Verification items for the finished model (mm, model axes). Face numbers are marked on the shaded views. A direction names the side the tool comes from. Round coordinates to 2 decimals unless told otherwise and drop trailing zeros. Loops run counter-clockwise (first coordinate to the right, second up) from the corner with the lowest first, then second, coordinate; pieces in that order, holes last. Notation, with made-up numbers: M -9.75,42.25 L 28.25,42.25 A36 ccw 28.25,81.25 Z; hole C 23,18.25 d5. An arc over 180 degrees is marked long. Answer as CSV lines item,"result".
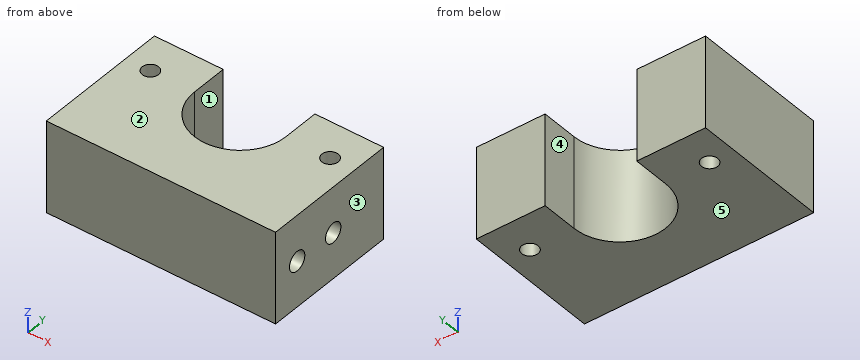
```python
from build123d import *

# Parameters (mm, degrees)
SKETCH1_W                 = 12.7
SKETCH1_H                 = 19.05
BASE_DEPTH                = 31.75
MOTORSLOT_DEPTH           = 40.144028919
MOTORHOLES_D              = 2.2606
F_6_32_TAPPED_HOLE1_D     = 2.7051
F_6_32_TAPPED_HOLE1_DEPTH = 8.382
F_6_32_TAPPED_HOLE1_TIP   = 0.81269403


with BuildPart() as part:
    # Sketch1 → Base (new body)
    with BuildSketch(Plane(origin=(0, 0, 0), x_dir=(0, 0, -1), z_dir=(1, 0, 0))):
        with Locations((6.35, 9.525)):
            Rectangle(SKETCH1_W, SKETCH1_H)
    extrude(amount=-BASE_DEPTH)

    # Sketch5 → MotorSlot (cut, through all)
    with BuildSketch(Plane(origin=(0, 0, -12.7), x_dir=(-1, 0, 0), z_dir=(0, 0, -1))):
        with BuildLine():
            Line((22.225, 19.05), (22.225, 13.97))
            ThreePointArc((22.225, 13.97), (15.875, 7.62), (9.525, 13.97))
            Line((9.525, 13.97), (9.525, 19.05))
            ThreePointArc((9.525, 19.05), (15.875, 25.4), (22.225, 19.05))
        make_face()
    extrude(amount=-MOTORSLOT_DEPTH, mode=Mode.SUBTRACT)

    # MotorHoles (through all)
    with Locations(Plane(origin=(0, 0, -12.7), x_dir=(-1, 0, 0), z_dir=(0, 0, -1))):
        with Locations((3.429, 13.97), (28.321, 13.97)):
            Hole(MOTORHOLES_D / 2)

    # #6-32 Tapped Hole1
    with Locations(Plane(origin=(0, 0, 0), x_dir=(0, 0, -1), z_dir=(1, 0, 0))):
        with Locations((6.35, 3.81), (6.35, 10.16)):
            Hole(F_6_32_TAPPED_HOLE1_D / 2, depth=F_6_32_TAPPED_HOLE1_DEPTH)
            with Locations((0, 0, -(F_6_32_TAPPED_HOLE1_DEPTH + F_6_32_TAPPED_HOLE1_TIP / 2))):  # 118° drill point
                Cone(0, F_6_32_TAPPED_HOLE1_D / 2, F_6_32_TAPPED_HOLE1_TIP, mode=Mode.SUBTRACT)


solid = part.part
```
1) Section check B-B (x = -6.5). Record the cut outline in (y, z).
Here are the results:
outline,"M 0,-12.7 L 19.05,-12.7 L 19.05,0 L 0,0 Z; hole C 3.81,-6.35 d2.71; hole C 10.16,-6.35 d2.71"
2) Section check C-C (x = -29). Record the cut outline in (y, z).
Here are the results:
outline,"M 0,-12.7 L 13.07,-12.7 L 13.07,0 L 0,0 Z; M 14.87,-12.7 L 19.05,-12.7 L 19.05,0 L 14.87,0 Z"
3) Section check D-D (x = -21). Record the cut outline in (y, z), plus the area to 3 significant figures.
Here are the results:
outline,"M 0,-12.7 L 10.22,-12.7 L 10.22,0 L 0,0 Z"
area,"130 mm^2"
4) Draft check along X on the marked faces 1, 2 and 3. Enter one of: +X half, -X half, draft (parallel to the pull), parting line (faces both ways), or undercut.
Here are the results:
face 1,"undercut"
face 2,"draft"
face 3,"+X half"
5) Section check A-A (z = -3.5). Record the cut outline in (x, y) (3 decimals), plus the area to 3 significant figures.
Here are the results:
outline,"M -31.75,0 L 0,0 L 0,19.05 L -9.525,19.05 L -9.525,13.97 A6.35 cw -22.225,13.97 L -22.225,19.05 L -31.75,19.05 Z; hole C -28.321,13.97 d2.261; hole C -3.429,13.97 d2.261"
area,"469 mm^2"
6) Material ranges on probe 1 along Y at (x, z) = (-2, -6.35); probe 2 along X at (y, z) = (16, -0.25) (3 decimals); probe 3 along Z at (x, y) = (-5.5, 3.75), recorded low to high.
Here are the results:
probe 1,"y = 0 to 2.46, 5.16 to 8.81, 11.51 to 19.05"
probe 2,"x = -31.75 to -22.225, -9.525 to 0"
probe 3,"z = -12.7 to -7.7, -5 to 0"
7) Set-up check for the marked faces 4 and 5: record each of +Z, -Z, +X, -X, +Y, -Y from which the full face is reachable in a straight line by a thin tool's end or side.
Here are the results:
face 4,"+Z, -Z, +Y"
face 5,"-Z, +X, -X, +Y, -Y"
8) Go/stop test with flat-tipped pins: pin 1 (1.5 mm diameter, centred on x = -13, z = -7, fed in from +Y); pin 2 (3 mm diameter, centred on x = -12.5, y = 15, fed in from +Z). Record where each tip stops, or that it passes through.
Here are the results:
pin 1,"stops at y = 8.76"
pin 2,"passes through"
